Geometry: final body of the model. Coordinates: model frame, mm. Face numbers are marked on the shaded views. Coordinates: 2 decimals unless noted, no trailing zeros. Loops run counter-clockwise (first coordinate to the right, second up) from the corner with the lowest first, then second, coordinate; pieces in that order, holes last. Notation, with made-up numbers: (71, 67.5) - (99, 67.5) arc R26 cw to (99, 88.5) - close; hole circle Ø11 at (-9, 20.5). An arc over 180 degrees is marked (long way). Answer in a Markdown table with one row per item.
from build123d import *

# Parameters (mm, degrees)
SKETCH1_W           = 220
SKETCH1_H           = 125
BOSS_EXTRUDE1_DEPTH = 20
SKETCH2_W           = 200
SKETCH2_H           = 105
CUT_EXTRUDE1_DEPTH  = 10
FILLET1_R           = 10
SKETCH3_W           = 171
SKETCH3_H           = 102.09
BOSS_EXTRUDE2_DEPTH = 5
SKETCH4_R           = 2
CUT_EXTRUDE2_DEPTH  = 129.962203765
SKETCH5_R           = 5
CUT_EXTRUDE3_DEPTH  = 5


with BuildPart() as part:
    # Sketch1 → Boss-Extrude1 (new body)
    with BuildSketch(Plane(origin=(0, 0, 0), x_dir=(1, 0, 0), z_dir=(0, 1, 0))):
        Rectangle(SKETCH1_W, SKETCH1_H)
    extrude(amount=BOSS_EXTRUDE1_DEPTH)

    # Sketch2 → Cut-Extrude1 (cut)
    with BuildSketch(Plane(origin=(0, 20, 0), x_dir=(1, 0, 0), z_dir=(0, 1, 0))):
        Rectangle(SKETCH2_W, SKETCH2_H)
    extrude(amount=-CUT_EXTRUDE1_DEPTH, mode=Mode.SUBTRACT)

    # Fillet1
    fillet1_edges = [part.edges().sort_by_distance(p)[0] for p in [
        (110, 20, 0),
        (0, 20, -62.5),
        (-110, 20, 0),
        (0, 20, 62.5),
    ]]
    fillet(fillet1_edges, radius=FILLET1_R - 0.0001)  # a hair under: the kernel refuses the full size

    # Sketch3 → Boss-Extrude2 (add)
    with BuildSketch(Plane.XZ):
        Rectangle(SKETCH3_W, SKETCH3_H)
    extrude(amount=BOSS_EXTRUDE2_DEPTH)

    # Sketch4 → Cut-Extrude2 (cut, through all)
    with BuildSketch(Plane.XZ.offset(5)):
        with Locations(Location((-65.5, 31.045, 0), (0, 0, 270))):
            Circle(SKETCH4_R)
        with Locations(Location((-65.5, -31.045, 0), (0, 0, 270))):
            Circle(SKETCH4_R)
        with Locations(Location((65.5, -31.045, 0), (0, 0, 270))):
            Circle(SKETCH4_R)
        with Locations(Location((65.5, 31.045, 0), (0, 0, 270))):
            Circle(SKETCH4_R)
    extrude(amount=-CUT_EXTRUDE2_DEPTH, mode=Mode.SUBTRACT)

    # Sketch5 → Cut-Extrude3 (cut)
    with BuildSketch(Plane(origin=(0, 10, 0), x_dir=(1, 0, 0), z_dir=(0, 1, 0))):
        with Locations(Location((-65.5, 31.045, 0), (0, 0, 270))):
            Circle(SKETCH5_R)
        with Locations(Location((-65.5, -31.045, 0), (0, 0, 270))):
            Circle(SKETCH5_R)
        with Locations(Location((65.5, -31.045, 0), (0, 0, 270))):
            Circle(SKETCH5_R)
        with Locations(Location((65.5, 31.045, 0), (0, 0, 270))):
            Circle(SKETCH5_R)
    extrude(amount=-CUT_EXTRUDE3_DEPTH, mode=Mode.SUBTRACT)


solid = part.part
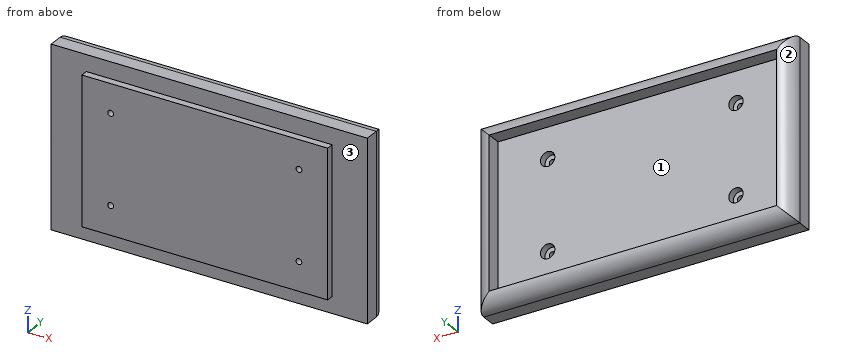
(1) First-contact query: pin 1 Ø6.5 at (x, z) = (-65.5, -31.045) entering from +Y; pin 2 Ø5.5 at (y, z) = (-3, 12.5) entering from -X; pin 3 Ø11 at (y, z) = (17, 4) entering from +X. Flat tips, straight axial feed; report the tip coordinate or a pass-through.
Verdict:
| item | result |
|---|---|
| pin 1 | stops at y = 5 |
| pin 2 | stops at x = -85.5 |
| pin 3 | stops at x = 109.89 |
(2) Ray query, probe 1 along X at (y, z) = (10.75, -34); probe 2 along Y at (x, z) = (-37, -12.5); probe 3 along Z at (x, y) = (-49.5, 17.75). Return the intervals inside material, ascending.
Verdict:
| item | result |
|---|---|
| probe 1 | x = -109.97 to -100, 100 to 109.97 |
| probe 2 | y = -5 to 10 |
| probe 3 | z = -58.82 to -52.5, 52.5 to 58.82 |
(3) Pull-direction query (X, two-part tool) for the marked faces 1, 2 and 3; classes: pulls with the +X half, pulls with the -X half, needs draft (parallel to the pull), parting line crosses it, or undercut.
Verdict:
| item | result |
|---|---|
| face 1 | undercut |
| face 2 | pulls with the -X half |
| face 3 | needs draft |
(4) Cut plane B-B on y = 16. Output: boundary loops of the cut face in (x, z).
Verdict:
| item | result |
|---|---|
| outline | (-108, -60.5) - (108, -60.5) - (108, 60.5) - (-108, 60.5) - close; hole (-100, -52.5) - (100, -52.5) - (100, 52.5) - (-100, 52.5) - close |
